Build history of the part. All positions in model axes, mm. Face numbers are marked on the shaded views. A direction names the side the tool comes from. Coordinates: 2 decimals unless noted, no trailing zeros. Order: outer loops, then holes, each group sorted by start corner. A loop starts at its lowest first (then second) coordinate and runs counter-clockwise, first axis right, second up. Notation, with made-up numbers: (71, 62) - (117, 62) arc R25 ccw to (117, 89) - close; hole circle Ø8 at (29.25, 72). An arc over 180 degrees is marked (long way). Write each question's results on one line, items separated by ' | '.
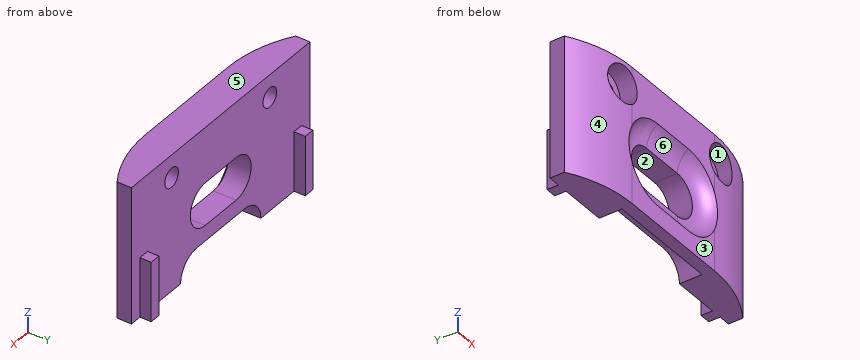
from build123d import *

# Parameters (mm, degrees)
EXTRUDE_1_DEPTH             = 24
SKETCH_2_W                  = 20
SKETCH_2_H                  = 4
CUT_EXTRUDE_1_DEPTH         = 4
SKETCH_3_W                  = 1.9
SKETCH_3_H                  = 10.472908188
EXTRUDE_2_DEPTH             = 2
FILLET_1_R                  = 4
CUT_EXTRUDE_2_DEPTH         = 34.690688625
SWEEP_START                 = -3.83
SWEEP_4_3_DEPTH             = 7.66
HOLE_WIZARD_M31_D           = 3.4
HOLE_WIZARD_M31_CBORE_D     = 6.5
HOLE_WIZARD_M31_CBORE_DEPTH = 3


with BuildPart() as part:
    # Эскиз1 → Бобышка-Вытянуть1 (new body)
    with BuildSketch(Plane.XY):
        with BuildLine():
            Line((-20.25, 2.586649223), (20.25, 2.586649223))
            Line((20.25, 2.586649223), (22.25, 2.586649223))
            Line((22.25, 2.586649223), (22.25, 0.053782912))
            ThreePointArc((22.25, 0.053782912), (16.495418641, -2.529195567), (10.25, -3.413350777))
            Line((10.25, -3.413350777), (-10.25, -3.413350777))
            ThreePointArc((-10.25, -3.413350777), (-16.495418641, -2.529195567), (-22.25, 0.053782912))
            Line((-22.25, 0.053782912), (-22.25, 2.586649223))
            Line((-22.25, 2.586649223), (-20.25, 2.586649223))
        make_face()
    extrude(amount=EXTRUDE_1_DEPTH)

    # Эскиз2 → Вырез-Вытянуть1 (cut)
    with BuildSketch(Plane(origin=(0, 2.586649223, 0), x_dir=(1, 0, 0), z_dir=(0, 1, 0))):
        with Locations((0, -2)):
            Rectangle(SKETCH_2_W, SKETCH_2_H)
    extrude(amount=-CUT_EXTRUDE_1_DEPTH, mode=Mode.SUBTRACT)

    # Эскиз3 → Бобышка-Вытянуть2 (add)
    with BuildSketch(Plane(origin=(0, 2.586649223, 0), x_dir=(1, 0, 0), z_dir=(0, 1, 0))):
        with Locations((19.2, -5.236454094)):
            Rectangle(SKETCH_3_W, SKETCH_3_H)
        with Locations((-19.2, -5.236454094)):
            Rectangle(SKETCH_3_W, SKETCH_3_H)
    extrude(amount=EXTRUDE_2_DEPTH)

    # Скругление1
    fillet_1_edges = [part.edges().sort_by_distance(p)[0] for p in [
        (-10, 0.586649223, 4),
        (10, 0.586649223, 4),
    ]]
    fillet(fillet_1_edges, radius=FILLET_1_R - 0.0001)  # a hair under: the kernel refuses the full size

    # Эскиз4 → Вырез-Вытянуть2 (cut, through all)
    with BuildSketch(Plane.XZ.offset(3.413350777)):
        with BuildLine():
            Line((-3.83, 14.25), (3.83, 14.25))
            ThreePointArc((3.83, 14.25), (7.58, 10.5), (3.83, 6.75))
            Line((3.83, 6.75), (-3.83, 6.75))
            ThreePointArc((-3.83, 6.75), (-7.58, 10.5), (-3.83, 14.25))
        make_face()
    extrude(amount=-CUT_EXTRUDE_2_DEPTH, mode=Mode.SUBTRACT)

    # Вырез-По траектории4: read off the stored shape, not the designer's step
    # Вырез-По траектории4 outline → Вырез-По траектории4 (revolve, cut)
    with BuildSketch(Plane(origin=(3.83, 0, 10.5), x_dir=(1, 0, 0), z_dir=(0, 0, 1))):
        with BuildLine():
            Line((3.75, -3.413351016), (7.214101753, -3.413351016))
            ThreePointArc((7.214101753, -3.413351016), (5.750000119, -1.949249231), (3.75, -1.413350777))
            Line((3.75, -1.413350777), (3.75, -3.413351016))
        make_face()
    revolve(axis=Axis((3.83, 0, 10.5), (0, 1, 0)), mode=Mode.SUBTRACT)

    # Sweep 4 2 outline → Sweep 4 2 (revolve, cut)
    with BuildSketch(Plane(origin=(-3.83, 0, 10.5), x_dir=(1, 0, 0), z_dir=(0, 0, 1))):
        with BuildLine():
            Line((3.75, -3.413350777), (7.214101615, -3.413350777))
            ThreePointArc((7.214101615, -3.413350777), (5.75, -1.949249162), (3.75, -1.413350777))
            Line((3.75, -1.413350777), (3.75, -3.413350777))
        make_face()
    revolve(axis=Axis((-3.83, 0, 10.5), (0, 1, 0)), mode=Mode.SUBTRACT)

    # Sweep 4 3 outline → Sweep 4 3 (cut)
    with BuildSketch(Plane.YZ.offset(SWEEP_START)):
        with BuildLine():
            ThreePointArc((-1.413350777, 14.25), (-1.949249162, 16.25), (-3.413350777, 17.714101615))
            Line((-3.413350777, 17.714101615), (-3.413350777, 3.285898385))
            ThreePointArc((-3.413350777, 3.285898385), (-1.949249162, 4.75), (-1.413350777, 6.75))
            Line((-1.413350777, 6.75), (-1.413350777, 14.25))
        make_face()
    extrude(amount=SWEEP_4_3_DEPTH, mode=Mode.SUBTRACT)

    # Цековка для винта с внутренним шестигранником M31 (through all)
    with Locations(Plane(origin=(-12.25, -3.413350777, 20), x_dir=(-1, 0, 0), z_dir=(0, -1, 0))):
        with Locations((0, 0), (-24.5, 0)):
            CounterBoreHole(HOLE_WIZARD_M31_D / 2, HOLE_WIZARD_M31_CBORE_D / 2, HOLE_WIZARD_M31_CBORE_DEPTH)


solid = part.part
1. Tool access for the marked faces 1, 2 and 3: list every direction of +Z, -Z, +X, -X, +Y, -Y with a clear straight run to the whole face (end or side of a thin tool).
Solved:
face 1: -Y | face 2: +Y, -Y | face 3: +Z, -Z, +X, -X, -Y
2. Two-plate mould, pull along X, no slides. Class the marked faces 4, 5 and 6: +X half, -X half, draft (parallel to the pull), parting line (faces both ways), or undercut.
Solved:
face 4: -X half | face 5: draft | face 6: undercut
3. Drop flat-ended pins along their axis: pin 1 Ø1.5 at (x, z) = (-17, 3.5) entering from +Y; pin 2 Ø4.5 at (x, y) = (1.5, 1) entering from -Z; pin 3 Ø2 at (x, z) = (13.5, 21.5) entering from -Y; pin 4 Ø2 at (x, y) = (19, 3.5) entering from +Z. Give the stop position or say it passes through.
Solved:
pin 1: stops at y = 2.59 | pin 2: stops at z = 4 | pin 3: stops at y = -0.41 | pin 4: stops at z = 24
4. Band-saw the part on D-D on x = -12.25. Give the cut face in (y, z).
Solved:
outline: (-3.32, 0) - (2.59, 0) - (2.59, 18.3) - (-0.41, 18.3) - (-0.41, 16.75) - (-3.32, 16.75) - close; (-3.32, 23.25) - (-0.41, 23.25) - (-0.41, 21.7) - (2.59, 21.7) - (2.59, 24) - (-3.32, 24) - close
5. Band-saw the part on B-B on z = 20. Give the cut face in (x, y).
Solved:
outline: (-22.25, 0.05) arc R22.5 ccw to (-15.5, -2.79) - (-15.5, -0.41) - (-13.95, -0.41) - (-13.95, 2.59) - (-22.25, 2.59) - close; (-10.55, -0.41) - (-9, -0.41) - (-9, -3.41) - (9, -3.41) - (9, -0.41) - (10.55, -0.41) - (10.55, 2.59) - (-10.55, 2.59) - close; (13.95, -0.41) - (15.5, -0.41) - (15.5, -2.79) arc R22.5 ccw to (22.25, 0.05) - (22.25, 2.59) - (13.95, 2.59) - close
6. Probe line 1 (X direction, y = 0.7, z = 20); line 2 (X direction, y = 3, z = 9.75); line 3 (Z direction, x = -12.25, y = 0.7). List the from-to ranges inside material, lowest first.
Solved:
line 1: x = -22.25 to -13.95, -10.55 to 10.55, 13.95 to 22.25 | line 2: x = -20.15 to -18.25, 18.25 to 20.15 | line 3: z = 0 to 18.3, 21.7 to 24
7. Band-saw the part on C-C on x = 3. Give the cut face in (y, z), then the cut area to 3 significant figures.
Solved:
outline: (-3.41, 0) - (-1.41, 0) - (-1.41, 4) - (2.59, 4) - (2.59, 6.75) - (-1.41, 6.75) arc R4 cw to (-3.41, 3.29) - close; (-3.41, 17.71) arc R4 cw to (-1.41, 14.25) - (2.59, 14.25) - (2.59, 24) - (-3.41, 24) - close | area: 73.2 mm2
8. Band-saw the part on A-A on y = 3.5. Give the cut face in (x, z).
Solved:
outline: (-20.15, 0) - (-18.25, 0) - (-18.25, 10.47) - (-20.15, 10.47) - close; (18.25, 0) - (20.15, 0) - (20.15, 10.47) - (18.25, 10.47) - close
